Design review of the part built by this model. Coordinates are the model's own, in mm. A direction names the side the tool comes from. Coordinates: 2 decimals unless noted, no trailing zeros. Loops run counter-clockwise (first coordinate to the right, second up) from the corner with the lowest first, then second, coordinate; pieces in that order, holes last. Notation, with made-up numbers: M 13,51 L 44,51 A14 ccw 44,71 Z; hole C 42,-12.5 d9. An arc over 180 degrees is marked long. Answer as a JSON object with one key per item and string values. Group by question number.
1. Insertion check: pin 1 (6 mm diameter, centred on y = 5, z = 140.5, fed in from +X); pin 2 (1 mm diameter, centred on x = 50, z = 141.5, fed in from +Y); pin 3 (1 mm diameter, centred on y = -59.5, z = 136, fed in from -X). Each pin has a flat end and moves straight along its axis. Give the tip position at first contact, or say it passes through.
2. Draft analysis for pull direction Y (two halves, no side actions). For faces 1 (the conical face through (-81.397, 74.639, 38.836)), 2 (the cylindrical face through (-55.55, -42.594, 95.978)), 3 (the flat face through (-37, -85, 139.283)), state which applies: +Y half, -Y half, draft (parallel to the pull), parting line (faces both ways), or undercut.
3. Consider section C-C (z = 66.5). State the section outline as (x, y) points, then the cut area to 3 significant figures.
4. To check wall thickness, follow probe 1 along Y at (x, z) = (0, -4); probe 2 along Z at (x, y) = (33.5, 84); probe 3 along Y at (x, z) = (-50, 60). State the ranges of each line that lie inside material, in increasing order.
5. Consider section A-A (y = 0). State the section outline as (x, z) points, then the cut area to 3 significant figures.
6. Consider section D-D (z = 145). State the section outline as (x, y) points.
7. Machinability: for faces 4 (the flat face through (-1, 1, 0)), 5 (the flat face through (1, 1, 175)), which of the approach directions +Z, -Z, +X, -X, +Y, -Y give a long, thin tool a straight path to every point of the face, cutting with its end or side? Answer none if there is none.
from build123d import *

# Parameters (mm, degrees)
SKETCH001_R    = 22.5
PAD_DEPTH      = 100
PAD_DEPTH_BACK = 40


with BuildPart() as part:
    # Sketch → Revolution (revolve)
    with BuildSketch(Plane.XZ):
        Polygon((70, 39.282857), (110, 39.282857), (117, 32.141428), (117, -7.858572), (110, -15), (50, -15), (50, 0), (0, 0), (0, 175), (50, 175), (70, 154.282857), align=None)
    revolve(axis=Axis((0, 0, 0), (0, 0, 1)))

    # Sketch001 (on Face1 of Revolution) → Pad (new body, two sides)
    with BuildSketch(Plane(origin=(0, 0, 39.282857), x_dir=(-1, 0, 0), z_dir=(0, 0, 1))) as pad_sk:
        with Locations((-37.5, 85)):
            Circle(SKETCH001_R)
        with Locations((37.5, 85)):
            Circle(SKETCH001_R)
    extrude(amount=PAD_DEPTH)
    extrude(pad_sk.sketch, amount=-PAD_DEPTH_BACK)


solid = part.part
Findings below:
{
 "1": {"pin 1": "stops at x = 69.97", "pin 2": "stops at y = 49.49", "pin 3": "stops at x = -37.67"},
 "2": {"face 1": "parting line", "face 2": "undercut", "face 3": "draft"},
 "3": {"outline": "C 0,0 d140; C -37.5,-85 d45; C 37.5,-85 d45", "area": "18,600 mm^2"},
 "4": {"probe 1": "y = -117 to -50, 50 to 117", "probe 2": "z = -15 to 39.28", "probe 3": "y = -103.71 to -66.29, -48.99 to 48.99"},
 "5": {"outline": "M -117,-7.86 L -110,-15 L -50,-15 L -50,0 L 50,0 L 50,-15 L 110,-15 L 117,-7.86 L 117,32.14 L 110,39.28 L 70,39.28 L 70,154.28 L 50,175 L -50,175 L -70,154.28 L -70,39.28 L -110,39.28 L -117,32.14 Z", "area": "29,700 mm^2"},
 "6": {"outline": "C 0,0 d140"},
 "7": {"face 4": "-Z", "face 5": "+Z, +X, -X, +Y, -Y"}
}
